Read the model definition and answer for the solid it produces. Units are mm, in the model's axes. Give positions to 0.01 mm unless a question says otherwise; leave off trailing zeros. Order: outer loops, then holes, each group sorted by start corner. A loop starts at its lowest first (then second) coordinate and runs counter-clockwise, first axis right, second up. Notation, with made-up numbers: (-13.75, -24.5) - (22.25, -24.5) arc R10 cw to (22.25, -5.5) - close; hole circle Ø4 at (36, 87.25). An arc over 180 degrees is marked (long way). Write each question's results on one line, items separated by ' | '.
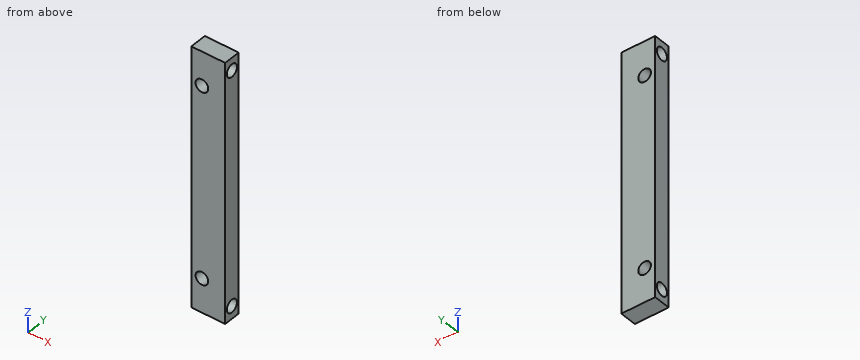
from build123d import *

# Parameters (mm, degrees)
F0_W     = 8
F0_H     = 65
F0_R     = 1.5
F1_DEPTH = 4
F2_R     = 1.5
F3_DEPTH = 25
F4_W     = 9.591324
F4_H     = 3.160866
F4_W_2   = 9.216423
F4_H_2   = 3.027778
F5_DEPTH = 25


with BuildPart() as f1:
    # F0 (on Front) → F1 (new body)
    with BuildSketch(Plane.XZ):
        with Locations((-4, 19.631475)):
            Rectangle(F0_W, F0_H)
        with Locations((-5.5, -2.868525)):
            Circle(F0_R, mode=Mode.SUBTRACT)
        with Locations((-5.5, 42.131475)):
            Circle(F0_R, mode=Mode.SUBTRACT)
    extrude(amount=F1_DEPTH)

    # F2 (on face) → F3 (cut)
    with BuildSketch(Plane.YZ):
        with Locations((-2, 47.131475)):
            Circle(F2_R)
        with Locations((-2, -7.868525)):
            Circle(F2_R)
    extrude(amount=-F3_DEPTH, mode=Mode.SUBTRACT)

    # F4 (on face) → F5 (cut)
    with BuildSketch(Plane.YZ):
        with Locations((-2.453811, 51.711908)):
            Rectangle(F4_W, F4_H)
        with Locations((-0.403113, -12.382414)):
            Rectangle(F4_W_2, F4_H_2)
    extrude(amount=-F5_DEPTH, mode=Mode.SUBTRACT)


solid = f1.part
(1) Section B-B (y = -2.6) is taken. Give the vertices of the cut face in (x, z).
Conclusion:
outline: (-8, -10.87) - (0, -10.87) - (0, -9.24) - (-8, -9.24) - close; (-8, -6.49) - (0, -6.49) - (0, 45.76) - (-8, 45.76) - close; (-8, 48.51) - (0, 48.51) - (0, 50.13) - (-8, 50.13) - close; hole circle Ø3 at (-5.5, -2.87); hole circle Ø3 at (-5.5, 42.13)
(2) Section A-A (x = -6.25) is taken. Give the vertices of the cut face in (y, z), plus the area to 3 significant figures.
Conclusion:
outline: (-4, -10.87) - (0, -10.87) - (0, -4.17) - (-4, -4.17) - close; (-4, -1.57) - (0, -1.57) - (0, 40.83) - (-4, 40.83) - close; (-4, 43.43) - (0, 43.43) - (0, 50.13) - (-4, 50.13) - close; hole circle Ø3 at (-2, -7.87); hole circle Ø3 at (-2, 47.13) | area: 209 mm^2
(3) Consider probe 1 along Z at (x, y) = (-2.5, -2); probe 2 along Z at (x, y) = (-5.5, -1.9); probe 3 along Z at (x, y) = (-5.5, -2.3). Determine where each line is inside the solid, lowest interval first. Write a range as [from, to].
Conclusion:
probe 1: [-10.87, -9.37], [-6.37, 45.63], [48.63, 50.13] | probe 2: [-10.87, -9.37], [-6.37, -4.37], [-1.37, 40.63], [43.63, 45.63], [48.63, 50.13] | probe 3: [-10.87, -9.34], [-6.4, -4.37], [-1.37, 40.63], [43.63, 45.66], [48.6, 50.13]
(4) This flat-tipped pin is pushed along its axis until it touches: pin 1 (2.5 mm diameter, centred on x = -5.5, z = -2.87, fed in from -Y). Where does it stop, or does it pass through?
Conclusion:
pin 1: through
(5) Section C-C (x = -2.5) is taken. Give the vertices of the cut face in (y, z).
Conclusion:
outline: (-4, -10.87) - (0, -10.87) - (0, 50.13) - (-4, 50.13) - close; hole circle Ø3 at (-2, -7.87); hole circle Ø3 at (-2, 47.13)
